Verification items for this drawing (mm, ordinates from the low corner). A direction names the side the tool comes from. Round coordinates to 2 decimals unless told otherwise and drop trailing zeros. Write each loop counter-clockwise with the first axis right and the second up, starting at its lowest first coordinate (ties: lowest second). Pieces come first, ordered by that corner, then holes. Notation, with made-up numbers: (6.5, -39.75) -> (53.5, -39.75) arc R27 ccw to (53.5, -5.75) -> close; hole circle Ø9 at (72, 10). An arc over 180 degrees is marked (long way). One line per item, written item: value.
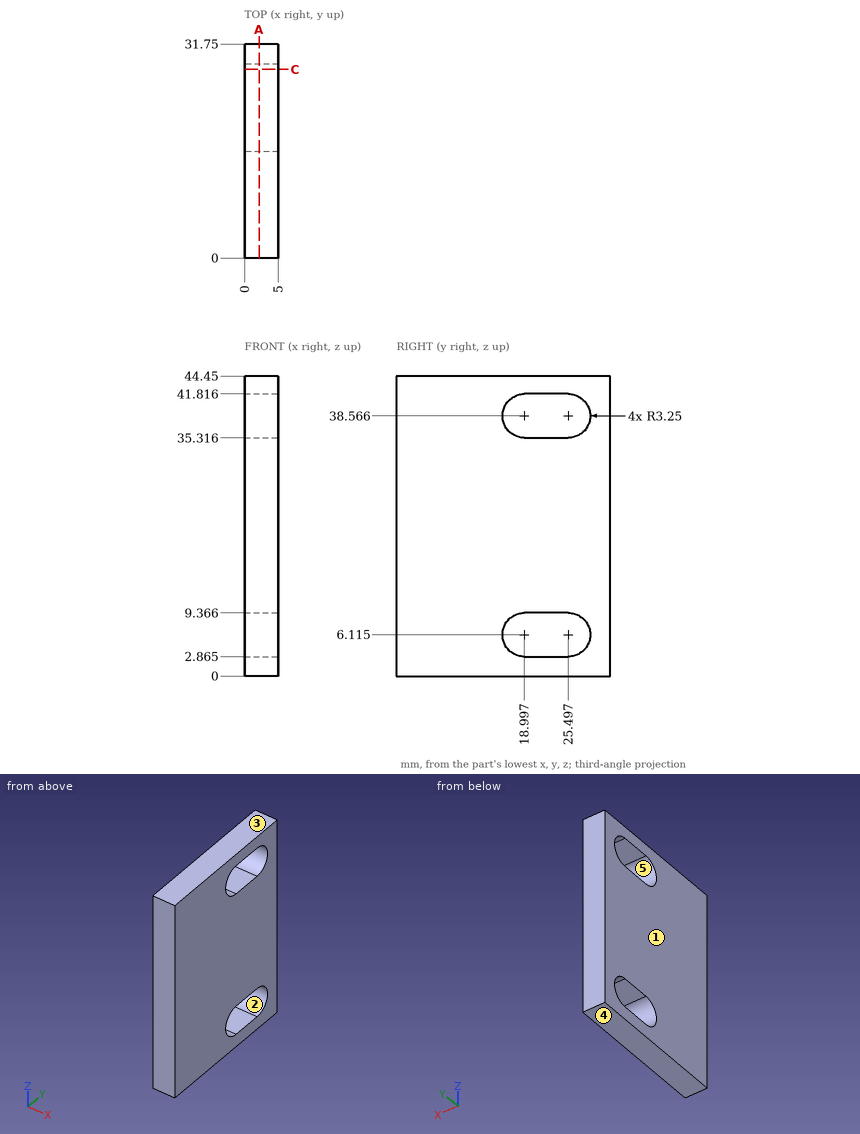
Item 1: Sectioned sample at C-C (y = 28). Enter the section's corners in (x, z).
Result set:
outline: (0, 0) -> (5, 0) -> (5, 4.04) -> (0, 4.04) -> close; (0, 8.19) -> (5, 8.19) -> (5, 36.49) -> (0, 36.49) -> close; (0, 40.64) -> (5, 40.64) -> (5, 44.45) -> (0, 44.45) -> close
Item 2: Release check for a two-part mould opening along Z. For the marked faces 1, 2 and 3 record: pulls with the +Z half, pulls with the -Z half, needs draft (parallel to the pull), parting line crosses it, or undercut.
Result set:
face 1: needs draft
face 2: undercut
face 3: pulls with the +Z half
Item 3: Material ranges on line 1 along Z through (x, y) = (1.7, 18), recorded low to high.
Result set:
line 1: 0 to 3.02, 9.21 to 35.47, 41.66 to 44.45
Item 4: Sectioned sample at A-A (x = 2.15). State how many separate pieces and enclosed holes the cut face has, then the cut area to 3 significant figures.
Result set:
separate pieces: 1
enclosed holes: 2
area: 1,260 mm^2
Item 5: Tool access check on the marked faces 4 and 5. Record the directions out of +Z, -Z, +X, -X, +Y, -Y that give a thin tool (end or side, any length) a straight path to the whole face; none if there is none.
Result set:
face 4: -Z, +X, -X, +Y, -Y
face 5: +X, -X
Item 6: Depth check by flat-ended pin: pin 1 (1.5 mm diameter, centred on x = 3, z = 17, fed in from -Y). Enter the tip coordinate at first touch or a pass-through.
Result set:
pin 1: y = 0
